```python
from build123d import *

# Parameters (mm, degrees)
SKETCH1_W            = 279.4
SKETCH1_H            = 101.6
BOSS_EXTRUDE1_DEPTH  = 6.35
SKETCH2_R            = 13.97
BOSS_EXTRUDE3_DEPTH  = 5.55625
SKETCH9_R            = 11.1125
CUT_EXTRUDE4_DEPTH   = 4.445
CUT_EXTRUDE5_START   = -5.55625
SKETCH10_R           = 11.1125
CUT_EXTRUDE5_DEPTH   = 5.55625
SKETCH11_R           = 7.9375
CUT_EXTRUDE6_DEPTH   = 285.078633923
SKETCH12_R           = 6.35
CUT_EXTRUDE7_DEPTH   = 285.051619429
SKETCH22_W           = 63.5
SKETCH22_H           = 63.5
BOSS_EXTRUDE7_DEPTH  = 12.7
SKETCH25_W           = 50.8
SKETCH25_H           = 50.8
CUT_EXTRUDE11_DEPTH  = 15.875
SKETCH32_R           = 4.7625
CUT_EXTRUDE12_DEPTH  = 6.35
SKETCH38_W           = 46.99
SKETCH38_H           = 18.470251096
CUT_EXTRUDE13_DEPTH  = 6.35
SKETCH60_R           = 4.7625
CUT_EXTRUDE23_DEPTH  = 6.35
SKETCH64_R           = 4.7625
CUT_EXTRUDE24_DEPTH  = 285.264471927
SKETCH69_W           = 33.02
SKETCH69_H           = 6.35
BOSS_EXTRUDE10_DEPTH = 19.05
SKETCH70_R           = 4.7625
SKETCH70_R_2         = 2.54
CUT_EXTRUDE26_DEPTH  = 6.35
SKETCH76_R           = 4.7625
CUT_EXTRUDE29_DEPTH  = 6.35
SKETCH77_W           = 46.99
SKETCH77_H           = 16.7871648
CUT_EXTRUDE30_DEPTH  = 6.35
SKETCH78_W           = 49.276
SKETCH78_H           = 66.342584104
CUT_EXTRUDE32_DEPTH  = 1.524
SKETCH79_R           = 4.7625
CUT_EXTRUDE33_DEPTH  = 4.826


with BuildPart() as part:
    # Sketch1 → Boss-Extrude1 (new body)
    with BuildSketch(Plane(origin=(0, 0, 0), x_dir=(1, 0, 0), z_dir=(0, 1, 0))):
        with Locations((-139.7, 0)):
            Rectangle(SKETCH1_W, SKETCH1_H)
    extrude(amount=BOSS_EXTRUDE1_DEPTH)

    # Sketch2 → Boss-Extrude3 (add)
    with BuildSketch(Plane(origin=(0, 6.35, 0), x_dir=(1, 0, 0), z_dir=(0, 1, 0))):
        with Locations(Location((-258.510557857, 0, 0), (0, 0, 90))):
            Circle(SKETCH2_R)
    extrude(amount=BOSS_EXTRUDE3_DEPTH)

    # Sketch9 → Cut-Extrude4 (cut)
    with BuildSketch(Plane(origin=(0, 11.90625, 0), x_dir=(1, 0, 0), z_dir=(0, 1, 0))):
        with Locations(Location((-258.510557857, 0, 0), (0, 0, 270))):
            Circle(SKETCH9_R)
    extrude(amount=-CUT_EXTRUDE4_DEPTH, mode=Mode.SUBTRACT)

    # Sketch10 → Cut-Extrude5 (cut)
    with BuildSketch(Plane(origin=(0, 0, 0), x_dir=(-1, 0, 0), z_dir=(0, -1, 0)).offset(CUT_EXTRUDE5_START)):
        with Locations(Location((258.510557857, 0, 0), (0, 0, 270))):
            Circle(SKETCH10_R)
    extrude(amount=CUT_EXTRUDE5_DEPTH, mode=Mode.SUBTRACT)

    # Sketch11 → Cut-Extrude6 (cut, through all)
    with BuildSketch(Plane(origin=(0, 7.46125, 0), x_dir=(1, 0, 0), z_dir=(0, 1, 0))):
        with Locations(Location((-258.510557857, 0, 0), (0, 0, 270))):
            Circle(SKETCH11_R)
    extrude(amount=-CUT_EXTRUDE6_DEPTH, mode=Mode.SUBTRACT)

    # Sketch12 → Cut-Extrude7 (cut, through all)
    with BuildSketch(Plane(origin=(0, 6.35, 0), x_dir=(1, 0, 0), z_dir=(0, 1, 0))):
        with Locations(Location((-134.666203771, 0, 0), (0, 0, 270))):
            Circle(SKETCH12_R)
    extrude(amount=-CUT_EXTRUDE7_DEPTH, mode=Mode.SUBTRACT)

    # Sketch22 → Boss-Extrude7 (add)
    with BuildSketch(Plane(origin=(0, 6.35, 0), x_dir=(1, 0, 0), z_dir=(0, 1, 0))):
        with Locations((-134.666203771, 0)):
            Rectangle(SKETCH22_W, SKETCH22_H)
    extrude(amount=BOSS_EXTRUDE7_DEPTH)

    # Sketch25 → Cut-Extrude11 (cut)
    with BuildSketch(Plane(origin=(0, 19.05, 0), x_dir=(1, 0, 0), z_dir=(0, 1, 0))):
        with Locations((-134.666203771, 0)):
            Rectangle(SKETCH25_W, SKETCH25_H)
    extrude(amount=-CUT_EXTRUDE11_DEPTH, mode=Mode.SUBTRACT)

    # Sketch32 → Cut-Extrude12 (cut)
    with BuildSketch(Plane(origin=(0, 6.35, 0), x_dir=(1, 0, 0), z_dir=(0, 1, 0))):
        with Locations(Location((-67.44195898, -40.64, 0), (0, 0, 270))):
            Circle(SKETCH32_R)
        with Locations(Location((-81.41195898, -40.64, 0), (0, 0, 270))):
            Circle(SKETCH32_R)
        with Locations(Location((-67.44195898, 40.64, 0), (0, 0, 270))):
            Circle(SKETCH32_R)
        with Locations(Location((-81.41195898, 40.64, 0), (0, 0, 270))):
            Circle(SKETCH32_R)
    extrude(amount=-CUT_EXTRUDE12_DEPTH, mode=Mode.SUBTRACT)

    # Sketch38 → Cut-Extrude13 (cut)
    with BuildSketch(Plane(origin=(0, 6.35, 0), x_dir=(1, 0, 0), z_dir=(0, 1, 0))):
        with Locations((-23.495, -24.777709652)):
            Rectangle(SKETCH38_W, SKETCH38_H)
    extrude(amount=-CUT_EXTRUDE13_DEPTH, mode=Mode.SUBTRACT)

    # Sketch60 → Cut-Extrude23 (cut)
    with BuildSketch(Plane(origin=(0, 6.35, 0), x_dir=(1, 0, 0), z_dir=(0, 1, 0))):
        with Locations(Location((-231.7492444, 41.324145444, 0), (0, 0, 270))):
            Circle(SKETCH60_R)
        with Locations(Location((-231.7492444, -39.369341378, 0), (0, 0, 270))):
            Circle(SKETCH60_R)
        with Locations(Location((-173.509244294, -39.369341378, 0), (0, 0, 270))):
            Circle(SKETCH60_R)
        with Locations(Location((-173.509244294, 41.324145444, 0), (0, 0, 270))):
            Circle(SKETCH60_R)
    extrude(amount=-CUT_EXTRUDE23_DEPTH, mode=Mode.SUBTRACT)

    # Sketch64 → Cut-Extrude24 (cut, through all)
    with BuildSketch(Plane(origin=(0, 6.35, 0), x_dir=(1, 0, 0), z_dir=(0, 1, 0))):
        with Locations(Location((-145.334203771, -41.275, 0), (0, 0, 270))):
            Circle(SKETCH64_R)
        with Locations(Location((-123.998203771, -41.275, 0), (0, 0, 270))):
            Circle(SKETCH64_R)
    cut_extrude24 = extrude(amount=-CUT_EXTRUDE24_DEPTH, mode=Mode.SUBTRACT)

    # Mirror1: Cut-Extrude24 across plane
    add(cut_extrude24.mirror(Plane.XY), mode=Mode.SUBTRACT)

    # Sketch69 → Boss-Extrude10 (add)
    with BuildSketch(Plane.XY.offset(50.8)):
        with Locations((-70.465355554, 3.175)):
            Rectangle(SKETCH69_W, SKETCH69_H)
    boss_extrude10 = extrude(amount=BOSS_EXTRUDE10_DEPTH)

    # Sketch70 → Cut-Extrude26 (cut)
    with BuildSketch(Plane(origin=(0, 6.35, 0), x_dir=(1, 0, 0), z_dir=(0, 1, 0))):
        with Locations(Location((-76.815355554, -60.325, 0), (0, 0, 270))):
            Circle(SKETCH70_R)
        with Locations(Location((-64.115355554, -60.325, 0), (0, 0, 270))):
            Circle(SKETCH70_R_2)
    cut_extrude26 = extrude(amount=-CUT_EXTRUDE26_DEPTH, mode=Mode.SUBTRACT)

    # Mirror2: Boss-Extrude10, Cut-Extrude26 across plane
    add(boss_extrude10.mirror(Plane.XY))
    add(cut_extrude26.mirror(Plane.XY), mode=Mode.SUBTRACT)

    # Sketch76 → Cut-Extrude29 (cut)
    with BuildSketch(Plane(origin=(0, 6.35, 0), x_dir=(1, 0, 0), z_dir=(0, 1, 0))):
        with Locations(Location((-264.668, 24.13, 0), (0, 0, 270))):
            Circle(SKETCH76_R)
        with Locations(Location((-252.222, 24.13, 0), (0, 0, 270))):
            Circle(SKETCH76_R)
    extrude(amount=-CUT_EXTRUDE29_DEPTH, mode=Mode.SUBTRACT)

    # Sketch77 → Cut-Extrude30 (cut)
    with BuildSketch(Plane(origin=(0, 6.35, 0), x_dir=(1, 0, 0), z_dir=(0, 1, 0))):
        with Locations((-23.495, -42.4064176)):
            Rectangle(SKETCH77_W, SKETCH77_H)
    extrude(amount=-CUT_EXTRUDE30_DEPTH, mode=Mode.SUBTRACT)

    # Sketch78 → Cut-Extrude32 (cut)
    with BuildSketch(Plane(origin=(0, 6.35, 0), x_dir=(1, 0, 0), z_dir=(0, 1, 0))):
        with Locations((-24.638, 17.628707948)):
            Rectangle(SKETCH78_W, SKETCH78_H)
    extrude(amount=-CUT_EXTRUDE32_DEPTH, mode=Mode.SUBTRACT)

    # Sketch79 → Cut-Extrude33 (cut)
    with BuildSketch(Plane(origin=(0, 4.826, 0), x_dir=(1, 0, 0), z_dir=(0, 1, 0))):
        with Locations(Location((-23.876, 15.191415896, 0), (0, 0, 270))):
            Circle(SKETCH79_R)
    extrude(amount=-CUT_EXTRUDE33_DEPTH, mode=Mode.SUBTRACT)


solid = part.part
```
Work out the finished part from the listing and answer in its coordinate system (mm). A direction names the side the tool comes from. Give positions to 0.01 mm unless a question says otherwise; leave off trailing zeros. Order: outer loops, then holes, each group sorted by start corner. A loop starts at its lowest first (then second) coordinate and runs counter-clockwise, first axis right, second up.
1. The mould has two halves that part along X. Classify faces 1 (the cylindrical face through (-266.26, 6.52, -1.72)), 2 (the flat face through (-102.916, 13, 0)), 3 (the flat face through (-71, 3, -69.85)): released by +X, released by -X, zero draft, split by the parting line, or undercut.
Result sheet:
face 1: undercut
face 2: released by +X
face 3: zero draft
2. Straight lines are drawn through the part: L1, parallel to Z at x = -82.5, y = 4; L2, parallel to X at y = 12.5, z = -8.5; L3, parallel to Y at x = -184, z = -15.5. For each, find the intervals that lie inside material, in ascending order.
Result sheet:
L1: z = -69.85 to -45.28, -36 to 36, 45.28 to 69.85
L2: x = -166.42 to -160.07, -109.27 to -102.92
L3: y = 0 to 6.35
3. Each of these flat-tipped pins is pushed along its axis until it touches: P1, Ø8, axis at y = 9, z = 40, coming from the +X side; P2, Ø1, axis at x = -111, y = 11.5, coming from the -Z side; P3, Ø8.5, axis at x = -124, z = -41.28, coming from the +Y side; P4, Ø7, axis at x = -188.5, y = 2.5, coming from the +Z side. Where does it stop, or does it pass through?
Result sheet:
P1: stops at x = -46.99
P2: stops at z = -31.75
P3: passes through
P4: stops at z = 50.8
4. Section B-B, the plane z = 40.64 is taken. Determine the outline of the cut face in (x, y).
Result sheet:
outline: (-279.4, 0) - (-236.34, 0) - (-236.34, 6.35) - (-279.4, 6.35) - close; (-227.16, 0) - (-178.1, 0) - (-178.1, 6.35) - (-227.16, 6.35) - close; (-168.92, 0) - (-150.05, 0) - (-150.05, 6.35) - (-168.92, 6.35) - close; (-140.61, 0) - (-128.72, 0) - (-128.72, 6.35) - (-140.61, 6.35) - close; (-119.28, 0) - (-86.17, 0) - (-86.17, 6.35) - (-119.28, 6.35) - close; (-76.65, 0) - (-72.2, 0) - (-72.2, 6.35) - (-76.65, 6.35) - close; (-62.68, 0) - (-46.99, 0) - (-46.99, 6.35) - (-62.68, 6.35) - close
5. Section A-A, the plane z = 0 is taken. Give the number of separate pieces and of enclosed holes in the cut face, and give its area (3 significant figures).
Result sheet:
separate pieces: 3
enclosed holes: 0
area: 1,560 mm2
6. For faces 4 (the flat face through (-135, 13, 31.75)), 5 (the flat face through (-135, 11, -25.4)), 6 (the flat face through (-166.416, 13, 0)), 7 (the flat face through (-24, 2, 15.543)), determine the directions among +Z, -Z, +X, -X, +Y, -Y from which every point of the face is accessible in a straight line to the end or side of a thin tool.
Result sheet:
face 4: +Z, +X, -X, +Y
face 5: +Y
face 6: +Z, -Z, +Y
face 7: +Z, +X, +Y, -Y
7. Section C-C, the plane x = -98 is taken. Determine the outline of the cut face in (y, z).
Result sheet:
outline: (0, -50.8) - (6.35, -50.8) - (6.35, 50.8) - (0, 50.8) - close
